Autodesk Inventor part; units mm, degrees
ref_plane "Work Plane2" through (14.2, -18.2, 10) normal (0, 0, 1) x (1, 0, 0)
ref_plane "Work Plane3" through (14.2, -18.2, 8) normal (0, 0, 1) x (1, 0, 0)
ref_plane "YZ Plane" through (0, 0, 0) normal (1, 0, 0) x (0, 1, 0)
ref_plane "Work Plane1" through (0, 185.6, 7) normal (0, 0, 1) x (1, 0, 0)
sketch "Sketch1" plane through (0, 185.6, 7) normal (0, 0, 1) x (1, 0, 0)
  circle A0 centre (-11.5, -11.5) radius 1
  circle A1 centre (11.5, 11.5) radius 1
  circle A2 centre (11.5, -11.5) radius 1
  circle A3 centre (-11.5, 11.5) radius 1
  circle A4 centre (0, 0) radius 11
  arc A5 (-14.2, -11.025) -> (-11.025, -14.2) centre (-11.025, -11.025) ccw
  line L0 (-11.025, -14.2) -> (11.025, -14.2)
  arc A6 (11.025, -14.2) -> (14.2, -11.025) centre (11.025, -11.025) ccw
  line L1 (14.2, -11.025) -> (14.2, 11.025)
  arc A7 (14.2, 11.025) -> (11.025, 14.2) centre (11.025, 11.025) ccw
  line L2 (11.025, 14.2) -> (-11.025, 14.2)
  arc A8 (-11.025, 14.2) -> (-14.2, 11.025) centre (-11.025, 11.025) ccw
  line L3 (-14.2, 11.025) -> (-14.2, -11.025)
  line L4 (-14.2, 14.2) -> (14.2, 14.2)
  line L5 (14.2, 14.2) -> (14.2, -14.2)
  line L6 (14.2, -14.2) -> (-14.2, -14.2)
  line L7 (-14.2, -14.2) -> (-14.2, 14.2)
  circle A9 centre (-11.5, 11.5) radius 1.6
  circle A10 centre (-11.5, -11.5) radius 1.624
  circle A11 centre (11.5, -11.5) radius 1.6374
  circle A12 centre (11.5, 11.5) radius 1.6
  line L8 (14.2, -14.2) -> (10.2, -14.2)
  line L9 (10.2, -14.2) -> (10.2, -34.2)
  line L10 (10.2, -34.2) -> (14.2, -34.2)
  line L11 (14.2, -34.2) -> (14.2, -14.2)
  circle A13 centre (0, 0) radius 12
  point P0 (0, -185.6)
  dimension "d0" = 3.2
  dimension "d3" = 4
  dimension "d4" = 20
  dimension "d25" = 1
ref_plane "Work Plane2" through (14.2, -18.2, 10) normal (0, 0, 1) x (1, 0, 0)
ref_plane "Work Plane3" through (14.2, -18.2, 8) normal (0, 0, 1) x (1, 0, 0)
extrude "Extrusion1" add sketch "Sketch1" along normal blind 5 contours L3 A8 L2 A7 L1 A6 L0 A5 | A5 L6 L7 | L7 L4 A8 | L0 L6 L11 L10 L9 | A6 L5 L6 | L4 L5 A7 | A9 | A10 | A11 | A12
sketch "Sketch2" plane through (10.2, 151.4, 7) normal (-1, 0, 0) x (0, 0, 1)
  line L0 (5, 20) -> (5, 0)
  line L1 (5, 0) -> (-5, 0)
  line L2 (-5, 0) -> (-5, 20)
  line L3 (-5, 20) -> (5, 20)
  line L4 (5, 20) -> (5, 0)
  point P0 (-7, -151.4)
  dimension "d30" = 10
extrude "Extrusion2" add sketch "Sketch2" against normal up to surface (4 mm away)
sketch "Sketch3" plane through (-14.2, 199.8, 12) normal (0, 0, 1) x (1, 0, 0)
  line L0 (28.4, 0) -> (37.4, 0)
  line L1 (37.4, 0) -> (37.4, -48.4)
  line L2 (37.4, -48.4) -> (28.4, -48.4)
  line L3 (28.4, -48.4) -> (28.4, 0)
  line L4 (34.9, -208) -> (31.9, -208)
  line L5 (34.9, -8) -> (34.9, -208)
  line L6 (31.9, -8) -> (34.9, -8)
  line L7 (31.9, -208) -> (31.9, -8)
  circle A0 centre (33.4, -25.7) radius 1.45
  circle A1 centre (33.4, -33.7) radius 1.45
  circle A2 centre (33.4, -41.7) radius 1.45
  circle A3 centre (33.4, -17.7) radius 1.45
  circle A4 centre (33.4, -25.7) radius 1.45
  circle A5 centre (33.4, -33.7) radius 1.45
  circle A6 centre (33.4, -9.7) radius 1.45
  circle A7 centre (33.4, -17.7) radius 1.45
  circle A8 centre (33.4, -25.7) radius 1.45
  circle A9 centre (14.2, -14.2) radius 12
  circle A10 centre (25.7, -25.7) radius 1
  circle A11 centre (2.7, -25.7) radius 1
  circle A12 centre (25.7, -2.7) radius 1
  circle A13 centre (2.7, -2.7) radius 1
  circle A14 centre (14.2, -14.2) radius 12
  line L8 (24.4, -48.4) -> (28.4, -48.4)
  line L9 (28.4, 0) -> (0, 0)
  line L10 (0, 0) -> (0, -28.4)
  line L11 (0, -28.4) -> (24.4, -28.4)
  line L12 (28.4, -48.4) -> (28.4, 0)
  line L13 (24.4, -28.4) -> (24.4, -48.4)
  point P0 (14.2, -199.8)
  dimension "d8" = 9
  dimension "d9" = 2.9
  dimension "d12" = 8
  dimension "d15" = 8
extrude "Extrusion3" add sketch "Sketch3" along normal blind 2 contours L0 L1 L2 L5 L6 L7 L3 | L3 L8 L13 L11 L10 L9 | L7 L6 L5 L2
sketch "Sketch4" plane through (-14.2, 199.8, 7) normal (0, 1, 0) x (1, 0, 0)
  line L0 (28.4, 0) -> (0, 0)
  line L1 (0, 0) -> (0, -7)
  line L2 (28.4, 0) -> (28.4, -5)
  line L3 (37.4, -7) -> (0, -7)
  line L4 (0, -7) -> (60, -7)
  line L5 (60, -7) -> (60, 5)
  line L6 (60, 5) -> (0, 5)
  line L7 (0, 5) -> (0, -7)
  line L8 (37.4, -7) -> (0, -7)
  line L9 (37.4, -5) -> (37.4, -7)
  line L10 (37.4, -5) -> (28.4, -5)
  line L11 (24.4, 5) -> (28.4, 5)
  point P0 (14.2, 7)
  dimension "d26" = 60
extrude "Extrusion4" add sketch "Sketch4" along normal blind 5
sketch "Sketch5" plane through (10.2, 151.4, 2) normal (-1, 0, 0) x (0, 0, 1)
  line L0 (0, 0) -> (12, 0)
  line L1 (12, 20) -> (12, 0)
  line L2 (5, 20) -> (12, 20)
  line L3 (0, 20) -> (5, 20)
  line L4 (0, 0) -> (0, 20)
  circle A0 centre (5, 15) radius 1.5
  circle A1 centre (5, 5) radius 1.5
  line L5 (10, 0) -> (10, 48.4)
  point P0 (-2, -151.4)
  dimension "d31" = 3
  dimension "d32" = 3
  dimension "d33" = 5
  dimension "d34" = 5
  dimension "d35" = 5
  dimension "d36" = 5
extrude "Extrusion5" cut sketch "Sketch5" against normal through all contours A0 | A1
sketch "Sketch6" plane through (-14.2, 171.4, 7) normal (-1, 0, 0) x (0, 0, 1)
  line L0 (0, 28.4) -> (0, 0)
  line L1 (0, 0) -> (7, 0)
  line L2 (7, 0) -> (7, 33.4)
  line L3 (-5, 33.4) -> (7, 33.4)
  line L4 (-5, 28.4) -> (-5, 33.4)
  line L5 (-5, 28.4) -> (0, 28.4)
  line L6 (7, 33.4) -> (-5, 33.4)
  line L7 (-5, 33.4) -> (-5, 0)
  line L8 (-5, 0) -> (7, 0)
  line L9 (7, 0) -> (7, 33.4)
  point P0 (-7, -171.4)
extrude "Extrusion6" add sketch "Sketch6" along normal blind 3
sketch "Sketch7" plane through (10.2, 171.4, 7) normal (0, -1, 0) x (1, 0, 0)
  line L0 (0, 0) -> (0, 7)
  line L1 (0, 7) -> (-27.4, 7)
  line L2 (-24.4, 0) -> (0, 0)
  line L3 (0, -5) -> (0, 0)
  line L4 (-27.4, 7) -> (0, 7)
  line L5 (0, 7) -> (0, -5)
  line L6 (0, -5) -> (-27.4, -5)
  line L7 (-27.4, -5) -> (-27.4, 7)
  line L8 (-27.4, -5) -> (-27.4, 7)
  line L9 (-24.4, -5) -> (-27.4, -5)
  line L10 (-24.4, -5) -> (-24.4, 0)
  point P0 (-10.2, -7)
extrude "Extrusion7" add sketch "Sketch7" along normal blind 3
sketch "Sketch8" plane through (-14.2, 204.8, 7) normal (0, 1, 0) x (1, 0, 0)
  line L0 (24.4, -1.5) -> (24.4, 1.5)
  circle A0 centre (55, 0) radius 1.5
  line L1 (60, -7) -> (60, 5)
  line L2 (60, 5) -> (-3, 5)
  circle A1 centre (45, 0) radius 1.5
  circle A2 centre (35, 0) radius 1.5
  point P0 (14.2, 7)
  point P1 (37.4, -5)
  dimension "d43" = 3
  dimension "d44" = 5
  dimension "d45" = 5
  dimension "d48" = 10
extrude "Extrusion8" cut sketch "Sketch8" against normal through all
sketch "Sketch9" plane through (45.8, 199.8, 2) normal (0, 0, -1) x (-1, 0, 0)
  line L0 (0, 0) -> (60, 0)
  line L1 (60, 0) -> (60, -28.4)
  line L2 (63, 5) -> (63, -31.4)
  line L3 (0, 5) -> (63, 5)
  line L4 (0, 0) -> (0, 5)
  line L5 (0, 5) -> (31.4076, 5)
  line L6 (31.4076, 5) -> (31.4076, -10)
  line L7 (31.4076, -10) -> (0, -10)
  line L8 (0, -10) -> (0, 5)
  line L9 (0, 0) -> (60, 0)
  circle A0 centre (26.4076, -5) radius 1.5
  circle A1 centre (20.4076, -5) radius 1.5
  circle A2 centre (14.4076, -5) radius 1.5
  circle A3 centre (8.4076, -5) radius 1.5
  circle A4 centre (2.4076, -5) radius 1.5
  line L10 (31.6, -28.4) -> (31.6, -48.4)
  line L11 (35.6, -48.4) -> (31.6, -48.4)
  line L12 (35.6, -48.4) -> (35.6, -31.4)
  line L13 (63, -31.4) -> (35.6, -31.4)
  line L14 (60, -28.4) -> (31.6, -28.4)
  point P0 (45.8, -199.8)
  dimension "d55" = 10
  dimension "d56" = 3
  dimension "d57" = 5
  dimension "d58" = 5
  dimension "d61" = 6
extrude "Extrusion9" add sketch "Sketch9" along normal blind 3
properties part number "30_CUBE_openXY_NEMA8mount"
Check sheet for the modelled part. Datum: model origin and axes. Units: mm. A direction names the side the tool comes from. Give positions to 0.01 mm unless a question says otherwise; leave off trailing zeros. Write each loop counter-clockwise with the first axis right and the second up, starting at its lowest first coordinate (ties: lowest second). Pieces come first, ordered by that corner, then holes. Notation, with made-up numbers: M -8.75,60 L 48.25,60 A26 cw 48.25,84 Z; hole C -39.75,31.25 d10. An arc over 180 degrees is marked long. Use one line per item in the form item = value.
(1) Section check C-C on z = 3.5. Record the boundary of the cut face in (x, y).
Answer block:
outline = M -17.2,168.4 L 10.2,168.4 L 10.2,151.4 L 14.2,151.4 L 14.2,171.4 L -14.2,171.4 L -14.2,199.8 L 45.8,199.8 L 45.8,204.8 L -17.2,204.8 Z
(2) Depth check by flat-ended pin: P1, Ø4.5, axis at x = -9.5, z = 9, coming from the -Y side; P2, Ø4, axis at x = 19.2, y = 182.1, coming from the -Z side; P3, Ø2.5, axis at x = 19.2, y = 190.1, coming from the +Z side; P4, Ø1.7, axis at x = 19.2, y = 166.1, coming from the +Z side. Enter the tip coordinate at first touch or a pass-through.
Answer block:
P1 = 168.4
P2 = 12
P3 = 2
P4 = through
(3) Section check A-A on z = 13.25. State how many separate pieces and enclosed holes the cut face has, plus the area to 3 significant figures.
Answer block:
separate_pieces = 1
enclosed_holes = 10
area = 1,310 mm2
(4) Material ranges on line 1 along Y through (x, z) = (19.2, 13); line 2 along X through (y, z) = (198, 11.5); line 3 along Y through (x, z) = (-8, 6.75), recorded low to high.
Answer block:
line_1 = 151.4 to 156.65, 159.55 to 164.65, 167.55 to 172.65, 175.55 to 180.65, 183.55 to 188.65, 191.55 to 204.8
line_2 = -17.2 to -11.94, -11.06 to 11.06, 11.94 to 14.2
line_3 = 168.4 to 171.4, 199.8 to 204.8
(5) Tool access check on faces 3 (the flat face through (-4, 168.4, 7)), 4 (the flat face through (23.2, 176, 13)), 5 (the cylindrical face through (18.886, 191.516, 12.986)). Record the directions out of +Z, -Z, +X, -X, +Y, -Y that give a thin tool (end or side, any length) a straight path to the whole face; none if there is none.
Answer block:
face_3 = +Z, -Z, -X, -Y
face_4 = +Z, +X, -Y
face_5 = +Z
(6) Section check B-B on x = 8. Record the boundary of the cut face in (y, z), plus the area to 3 significant figures.
Answer block:
outline = M 168.4,-1 L 171.4,-1 L 171.4,7 L 176.66,7 L 176.66,14 L 168.4,14 Z; M 194.54,7 L 199.8,7 L 199.8,-1 L 204.8,-1 L 204.8,14 L 194.54,14 Z
area = 194 mm2
(7) Draft check along Z on faces 1 (the cylindrical face through (20.475, 202.335, 8.464)), 2 (the cylindrical face through (18.886, 159.516, 12.986)). Enter one of: pulls with the +Z half, pulls with the -Z half, needs draft (parallel to the pull), parting line crosses it, or undercut.
Answer block:
face_1 = undercut
face_2 = needs draft
